Autodesk Inventor part; units mm, degrees
ref_plane "S1_XY" through (0, -1.5, 0) normal (-1, 0, 0) x (0, 0, -1)
ref_plane "S1_YZ" through (0, -1.5, 0) normal (0, 0, -1) x (0, -1, 0)
ref_plane "S1_ZX" through (0, -1.5, 0) normal (0, -1, 0) x (-1, 0, 0)
ref_plane "S1_XY" through (0, -1.5, 0) normal (-1, 0, 0) x (0, 0, -1)
ref_plane "S1_YZ" through (0, -1.5, 0) normal (0, 0, -1) x (0, -1, 0)
ref_plane "S1_ZX" through (0, -1.5, 0) normal (0, -1, 0) x (-1, 0, 0)
ref_plane "S2_XY" through (200, -1.5, 0) normal (1, 0, 0) x (0, 0, -1)
ref_plane "S2_YZ" through (200, -1.5, 0) normal (0, 0, -1) x (0, 1, 0)
ref_plane "S2_ZX" through (200, -1.5, 0) normal (0, 1, 0) x (1, 0, 0)
sketch "Sketch_1" plane through (0, 0, 0) normal (1, 0, 0) x (0, 1, 0)
  arc A0 (2.073, 16.9448) -> (-1.5, 14) centre (1.5, 14) ccw
  line L0 (-1.5, 14) -> (-1.5, -14)
  arc A1 (-1.5, -14) -> (2.073, -16.9448) centre (1.5, -14) ccw
  line L1 (2.073, -16.9448) -> (11.373, -15.1352)
  arc A2 (11.373, -15.1352) -> (13.8, -12.1904) centre (10.8, -12.1904) ccw
  line L2 (13.8, -12.1904) -> (13.8, -8.25)
  line L3 (13.8, -8.25) -> (12.3, -8.25)
  line L4 (12.3, -8.25) -> (12.3, -12.1904)
  arc A3 (11.0865, -13.6628) -> (12.3, -12.1904) centre (10.8, -12.1904) ccw
  line L5 (11.0865, -13.6628) -> (1.7865, -15.4724)
  arc A4 (0, -14) -> (1.7865, -15.4724) centre (1.5, -14) ccw
  line L6 (0, -14) -> (0, 14)
  arc A5 (1.7865, 15.4724) -> (0, 14) centre (1.5, 14) ccw
  line L7 (1.7865, 15.4724) -> (11.0865, 13.6628)
  arc A6 (12.3, 12.1904) -> (11.0865, 13.6628) centre (10.8, 12.1904) ccw
  line L8 (12.3, 12.1904) -> (12.3, 8.25)
  line L9 (12.3, 8.25) -> (13.8, 8.25)
  line L10 (13.8, 8.25) -> (13.8, 12.1904)
  arc A7 (13.8, 12.1904) -> (11.373, 15.1352) centre (10.8, 12.1904) ccw
  line L11 (11.373, 15.1352) -> (2.073, 16.9448)
extrude "Extrusion1" add sketch "Sketch_1" along normal blind 200 and the other way blind 100
sketch "Sketch2" plane through (-100, -1.5, -14) normal (0, -1, 0) x (1, 0, 0)
  circle A0 centre (26.56, 10.8287) radius 19.7262
  point P0 (100, 14)
sketch "草图3" plane through (200, -1.5, -14) normal (0, -1, 0) x (1, 0, 0)
  circle A0 centre (-27.2013, 14) radius 12.4918
  point P0 (-200, 14)
sketch "草图4" plane through (-100, 0, 0) normal (-1, 0, 0) x (0, 0, 1)
  circle A0 centre (11.9436, 5.123) radius 5.6638
  point P0 (0, 0)
properties part number "3932-200"
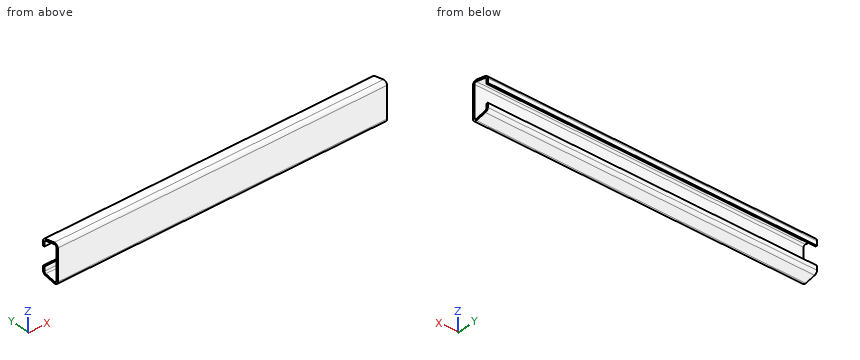
The listing builds one solid part. Answer for the finished solid, in the listing's coordinates (mm). Give positions to 0.01 mm unless a question says otherwise; leave off trailing zeros. Loops run counter-clockwise (first coordinate to the right, second up) from the corner with the lowest first, then second, coordinate; pieces in that order, holes last.
Item 1: Each of these flat-tipped pins is pushed along its axis until it touches: pin 1 Ø1 at (x, y) = (79, 4) entering from +Z; pin 2 Ø3 at (x, y) = (-41, 11.5) entering from -Z; pin 3 Ø1.2 at (x, y) = (94.5, 13) entering from -Z. Where does it stop, or does it pass through?
Derived:
pin 1: stops at z = 16.67
pin 2: stops at z = -15.4
pin 3: stops at z = -14.73
Item 2: Find the intervals of material crossed by line 1 along Y through (x, z) = (26.5, 11); line 2 along Y through (x, z) = (151.5, 2); line 3 along Z through (x, y) = (60.5, 2), in increasing order.
Derived:
line 1: y = -1.5 to 0, 12.3 to 13.8
line 2: y = -1.5 to 0
line 3: z = -16.96 to -15.43, 15.43 to 16.96
Item 3: A cutting plane is placed at A-A (y = 4.5). Give the vertices of the cut face in (x, z), then the cut area to 3 significant figures.
Derived:
outline: (-100, -16.47) - (200, -16.47) - (200, -14.94) - (-100, -14.94) - close; (-100, 14.94) - (200, 14.94) - (200, 16.47) - (-100, 16.47) - close
area: 917 mm2
Item 4: A cutting plane is placed at B-B (x = -15). Give the vertices of the cut face in (y, z), then the cut area to 3 significant figures.
Derived:
outline: (-1.5, -14) arc R3 ccw to (2.07, -16.94) - (11.37, -15.14) arc R3 ccw to (13.8, -12.19) - (13.8, -8.25) - (12.3, -8.25) - (12.3, -12.19) arc R1.5 cw to (11.09, -13.66) - (1.79, -15.47) arc R1.5 cw to (0, -14) - (0, 14) arc R1.5 cw to (1.79, 15.47) - (11.09, 13.66) arc R1.5 cw to (12.3, 12.19) - (12.3, 8.25) - (13.8, 8.25) - (13.8, 12.19) arc R3 ccw to (11.37, 15.14) - (2.07, 16.94) arc R3 ccw to (-1.5, 14) - close
area: 103 mm2
